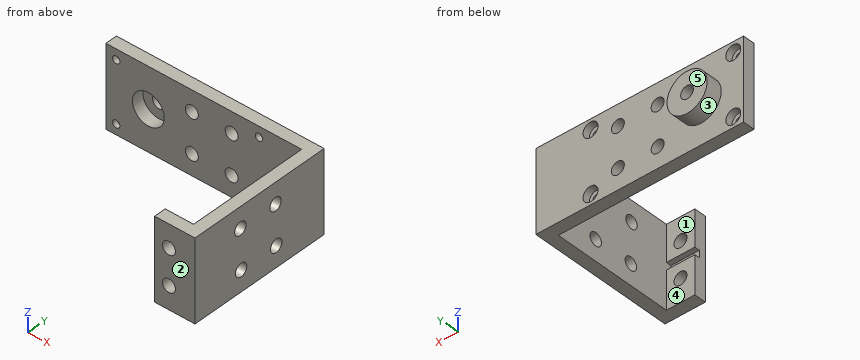
```python
from build123d import *

# Parameters (mm, degrees)
SKETCH1_W           = 52.25
SKETCH1_H           = 20.5
BOSS_EXTRUDE1_DEPTH = 3
SKETCH2_W           = 3
SKETCH2_H           = 20.5
BOSS_EXTRUDE2_DEPTH = 33.75
SKETCH3_W           = 20.5
SKETCH3_H           = 3
BOSS_EXTRUDE3_DEPTH = 7.15
SKETCH4_R           = 1.625
CUT_EXTRUDE1_DEPTH  = 3
SKETCH5_W           = 1.8
SKETCH5_H           = 1.3
CUT_EXTRUDE2_DEPTH  = 7.15
SKETCH6_R           = 1.625
CUT_EXTRUDE3_DEPTH  = 3
SKETCH7_R           = 1.625
CUT_EXTRUDE4_DEPTH  = 3
SKETCH8_R           = 1.875
CUT_EXTRUDE5_DEPTH  = 1.75
SKETCH9_R           = 0.925
CUT_EXTRUDE6_DEPTH  = 1.25
SKETCH12_R          = 5.05
BOSS_EXTRUDE4_DEPTH = 4
SKETCH11_R          = 4
CUT_EXTRUDE7_DEPTH  = 3
SKETCH13_R          = 1.6
CUT_EXTRUDE8_DEPTH  = 4


with BuildPart() as part:
    # Sketch1 → Boss-Extrude1 (new body)
    with BuildSketch(Plane(origin=(0, 0, 0), x_dir=(1, 0, 0), z_dir=(0, 1, 0))):
        Rectangle(SKETCH1_W, SKETCH1_H)
    extrude(amount=-BOSS_EXTRUDE1_DEPTH)

    # Sketch2 → Boss-Extrude2 (add)
    with BuildSketch(Plane.XZ.offset(3)):
        with Locations((24.625, 0)):
            Rectangle(SKETCH2_W, SKETCH2_H)
    extrude(amount=BOSS_EXTRUDE2_DEPTH)

    # Sketch3 → Boss-Extrude3 (add)
    with BuildSketch(Plane.ZY.offset(-23.125)):
        with Locations((0, -35.25)):
            Rectangle(SKETCH3_W, SKETCH3_H)
    extrude(amount=BOSS_EXTRUDE3_DEPTH)

    # Sketch4 → Cut-Extrude1 (cut)
    with BuildSketch(Plane.XZ.offset(36.75)):
        with Locations((19.575, 4.475)):
            Circle(SKETCH4_R)
        with Locations((19.575, -4.475)):
            Circle(SKETCH4_R)
    extrude(amount=-CUT_EXTRUDE1_DEPTH, mode=Mode.SUBTRACT)

    # Sketch5 → Cut-Extrude2 (cut)
    with BuildSketch(Plane.ZY.offset(-15.975)):
        with Locations((0.235327499, -34.4)):
            Rectangle(SKETCH5_W, SKETCH5_H)
    extrude(amount=-CUT_EXTRUDE2_DEPTH, mode=Mode.SUBTRACT)

    # Sketch6 → Cut-Extrude3 (cut)
    with BuildSketch(Plane.ZY.offset(-23.125)):
        with Locations((-4.997772224, -13.625)):
            Circle(SKETCH6_R)
        with Locations((-4.997772224, -23.625)):
            Circle(SKETCH6_R)
        with Locations((5, -23.836070013)):
            Circle(SKETCH6_R)
        with Locations((5, -13.836070013)):
            Circle(SKETCH6_R)
    extrude(amount=-CUT_EXTRUDE3_DEPTH, mode=Mode.SUBTRACT)

    # Sketch7 → Cut-Extrude4 (cut)
    with BuildSketch(Plane(origin=(0, 0, 0), x_dir=(1, 0, 0), z_dir=(0, 1, 0))):
        with Locations((-4.5, 5)):
            Circle(SKETCH7_R)
        with Locations((-4.5, -5)):
            Circle(SKETCH7_R)
        with Locations((5.5, 5)):
            Circle(SKETCH7_R)
        with Locations((5.5, -5)):
            Circle(SKETCH7_R)
    extrude(amount=-CUT_EXTRUDE4_DEPTH, mode=Mode.SUBTRACT)

    # Sketch8 → Cut-Extrude5 (cut)
    with BuildSketch(Plane(origin=(0, 0, 0), x_dir=(1, 0, 0), z_dir=(0, 1, 0))):
        with Locations((-23.525, 7.65)):
            Circle(SKETCH8_R)
        with Locations((-23.525, -7.65)):
            Circle(SKETCH8_R)
        with Locations((12.375, 7.65)):
            Circle(SKETCH8_R)
        with Locations((12.375, -7.65)):
            Circle(SKETCH8_R)
    extrude(amount=-CUT_EXTRUDE5_DEPTH, mode=Mode.SUBTRACT)

    # Sketch9 → Cut-Extrude6 (cut)
    with BuildSketch(Plane(origin=(0, -1.75, 0), x_dir=(1, 0, 0), z_dir=(0, 1, 0))):
        with Locations((-23.525, 7.65)):
            Circle(SKETCH9_R)
        with Locations((-23.525, -7.65)):
            Circle(SKETCH9_R)
        with Locations((12.375, -7.65)):
            Circle(SKETCH9_R)
        with Locations((12.375, 7.65)):
            Circle(SKETCH9_R)
    extrude(amount=-CUT_EXTRUDE6_DEPTH, mode=Mode.SUBTRACT)

    # Sketch12 → Boss-Extrude4 (add)
    with BuildSketch(Plane(origin=(0, 0, 0), x_dir=(1, 0, 0), z_dir=(0, 1, 0))):
        with Locations((-15.442849896, 0)):
            Circle(SKETCH12_R)
    extrude(amount=BOSS_EXTRUDE4_DEPTH)

    # Sketch11 → Cut-Extrude7 (cut)
    with BuildSketch(Plane.XZ.offset(3)):
        with Locations((-15.442849896, 0)):
            Circle(SKETCH11_R)
    extrude(amount=-CUT_EXTRUDE7_DEPTH, mode=Mode.SUBTRACT)

    # Sketch13 → Cut-Extrude8 (cut)
    with BuildSketch(Plane.XZ):
        with Locations((-15.442849896, 0)):
            Circle(SKETCH13_R)
    extrude(amount=-CUT_EXTRUDE8_DEPTH, mode=Mode.SUBTRACT)


solid = part.part
```
Check sheet for the modelled part. Datum: model origin and axes. Units: mm. Face numbers are marked on the shaded views. A direction names the side the tool comes from. Coordinates: 2 decimals unless noted, no trailing zeros. Write each loop counter-clockwise with the first axis right and the second up, starting at its lowest first coordinate (ties: lowest second). Pieces come first, ordered by that corner, then holes. Notation, with made-up numbers: M -23.75,-0.75 L 0.25,-0.75 A15 ccw 0.25,23.25 Z; hole C -39,29.25 d4. An arc over 180 degrees is marked long. Use one line per item in the form item = value.
Item 1: Sectioned sample at C-C, the plane x = -4. Record the cut outline in (y, z).
Answer below:
outline = M -3,-10.25 L 0,-10.25 L 0,-6.55 L -3,-6.55 Z; M -3,-3.45 L 0,-3.45 L 0,3.45 L -3,3.45 Z; M -3,6.55 L 0,6.55 L 0,10.25 L -3,10.25 Z
Item 2: Sectioned sample at A-A, the plane z = 0. Record the cut outline in (x, y) (3 decimals).
Answer below:
outline = M -26.125,-3 L -19.443,-3 L -19.443,0 L -17.043,0 L -17.043,4 L -20.493,4 L -20.493,0 L -26.125,0 Z; M -13.843,0 L -11.443,0 L -11.443,-3 L 23.125,-3 L 23.125,-35.05 L 15.975,-35.05 L 15.975,-36.75 L 26.125,-36.75 L 26.125,0 L -10.393,0 L -10.393,4 L -13.843,4 Z
Item 3: Sectioned sample at D-D, the plane y = -10. Record the cut outline in (x, z) (3 decimals).
Answer below:
outline = M 23.125,-10.25 L 26.125,-10.25 L 26.125,10.25 L 23.125,10.25 Z
Item 4: Release check for a two-part mould opening along Y. For the marked faces 1, 2 and 3 record: pulls with the +Y half, pulls with the -Y half, needs draft (parallel to the pull), parting line crosses it, or undercut.
Answer below:
face_1 = undercut
face_2 = pulls with the -Y half
face_3 = needs draft
Item 5: Gauge pin test, flat ends, axial feed: pin 1 Ø3 at (x, z) = (-16.5, -2.5) entering from -Y; pin 2 Ø3 at (x, z) = (-15.44, 0) entering from +Y; pin 3 Ø12 at (x, z) = (19, -6.5) entering from +Y; pin 4 Ø3 at (y, z) = (-30.5, 5.5) entering from -X (3 decimals). Record the tip position at first contact, or that the pin passes through.
Answer below:
pin_1 = -3
pin_2 = through
pin_3 = 0
pin_4 = 23.125
Item 6: Set-up check for the marked faces 4 and 5: record each of +Z, -Z, +X, -X, +Y, -Y from which the full face is reachable in a straight line by a thin tool's end or side.
Answer below:
face_4 = +Z, -Z, -X
face_5 = +Z, -Z, +X, -X, +Y
Item 7: Material ranges on L1, parallel to X at y = -2.1, z = 7.65 (3 decimals); L2, parallel to Y at x = 25.35, z = 5; L3, parallel to Y at x = -8.5, z = 7.5, recorded low to high. Write a range as from..to.
Answer below:
L1 = -26.125..-24.45, -22.6..11.45, 13.3..26.125
L2 = -36.75..-25.46, -22.21..-15.46, -12.21..0
L3 = -3..0
Item 8: Sectioned sample at B-B, the plane z = 7.65. Record the cut outline in (x, y) (3 decimals).
Answer below:
outline = M -26.125,-3 L -24.45,-3 L -24.45,-1.75 L -25.4,-1.75 L -25.4,0 L -26.125,0 Z; M -22.6,-3 L 11.45,-3 L 11.45,-1.75 L 10.5,-1.75 L 10.5,0 L -21.65,0 L -21.65,-1.75 L -22.6,-1.75 Z; M 13.3,-3 L 23.125,-3 L 23.125,-33.75 L 15.975,-33.75 L 15.975,-36.75 L 26.125,-36.75 L 26.125,0 L 14.25,0 L 14.25,-1.75 L 13.3,-1.75 Z
